Could you check a few things on this drawing? It's one solid part, dimensions in mm from its lowest x, y, z. A direction names the side the tool comes from. Give positions to 0.01 mm unless a question says otherwise; leave off trailing zeros. Order: outer loops, then holes, each group sorted by start corner. A loop starts at its lowest first (then second) coordinate and runs counter-clockwise, first axis right, second up. Notation, with made-up numbers: (7.5, 60) -> (22.5, 60) arc R33 cw to (22.5, 91) -> close; hole circle Ø4 at (-38.5, -36). An arc over 180 degrees is marked (long way). Answer as CSV lines item,"result".
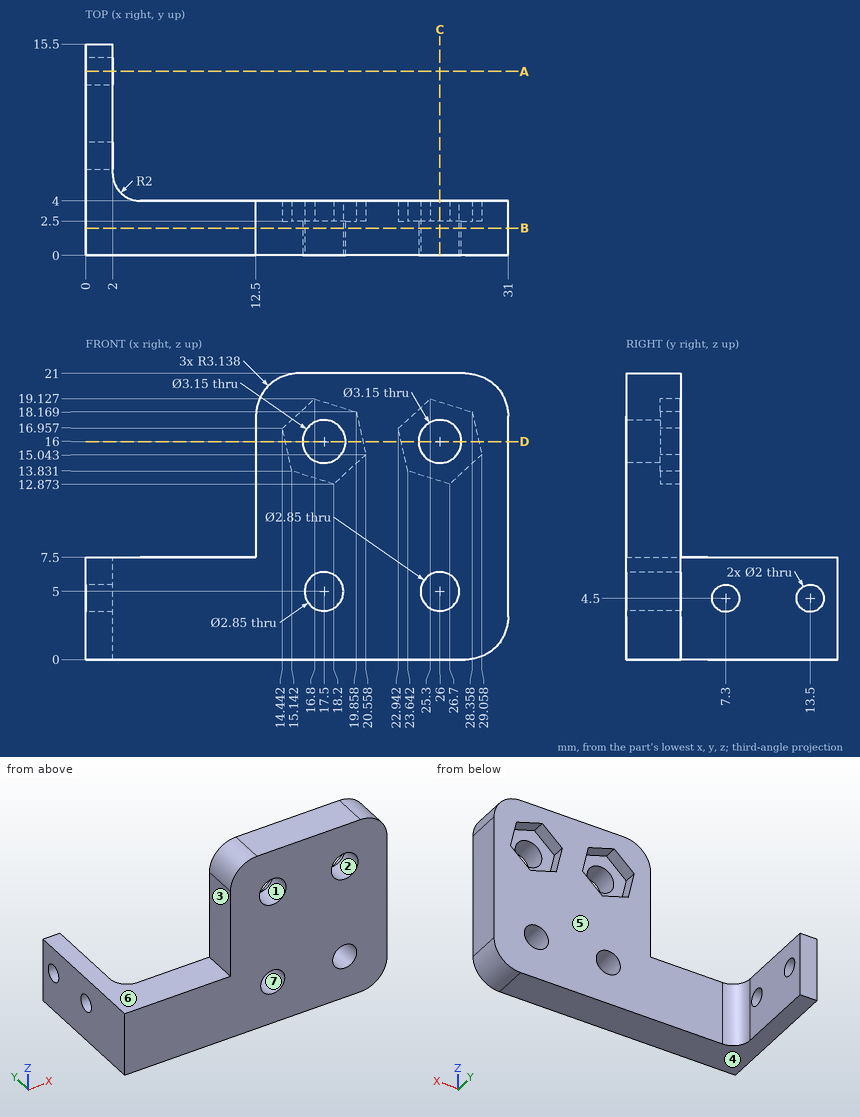
Item 1: Imagine slicing it at D-D, the plane z = 16. Please give me the cut outline in (x, y) (1 decimal).
Numbers:
outline,"(12.5, 0) -> (15.9, 0) -> (15.9, 2.5) -> (14.7, 2.5) -> (14.7, 4) -> (12.5, 4) -> close; (19.1, 0) -> (24.4, 0) -> (24.4, 2.5) -> (23.2, 2.5) -> (23.2, 4) -> (20.3, 4) -> (20.3, 2.5) -> (19.1, 2.5) -> close; (27.6, 0) -> (31, 0) -> (31, 4) -> (28.8, 4) -> (28.8, 2.5) -> (27.6, 2.5) -> close"
Item 2: Please list where these lines run through material, in increasing order: line 1 along Z through (x, y) = (17.5, 1.2) (1 decimal); line 2 along Z through (x, y) = (0.45, 7.3); line 3 along Z through (x, y) = (27, 1.25) (1 decimal).
Numbers:
line 1,"z = 0 to 3.6, 6.4 to 14.4, 17.6 to 21"
line 2,"z = 0 to 3.5, 5.5 to 7.5"
line 3,"z = 0 to 4, 6 to 14.8, 17.2 to 21"
Item 3: Imagine slicing it at B-B, the plane y = 2. Give the number of separate pieces and of enclosed holes in the cut face.
Numbers:
separate pieces,"1"
enclosed holes,"4"
Item 4: For pin 1 (5 mm diameter, centred on x = 15, z = 14.5, fed in from -Y); pin 2 (1.5 mm diameter, centred on x = 22, z = 18, fed in from +Y); pin 3 (1.2 mm diameter, centred on y = 1.5, z = 11, fed in from -X); pin 4 (2 mm diameter, centred on y = 12, z = 4, fed in from +X), each with a flat end and sliding along its axis, tell me the tip position at first contact or that it passes through.
Numbers:
pin 1,"stops at y = 0"
pin 2,"stops at y = 4"
pin 3,"stops at x = 12.5"
pin 4,"stops at x = 2"
Item 5: Imagine slicing it at C-C, the plane x = 26. Please give me the cut outline in (y, z) (1 decimal).
Numbers:
outline,"(0, 0) -> (4, 0) -> (4, 3.6) -> (0, 3.6) -> close; (0, 6.4) -> (4, 6.4) -> (4, 13.1) -> (2.5, 13.1) -> (2.5, 14.4) -> (0, 14.4) -> close; (0, 17.6) -> (2.5, 17.6) -> (2.5, 18.9) -> (4, 18.9) -> (4, 21) -> (0, 21) -> close"
Item 6: Imagine slicing it at A-A, the plane y = 13.5. Please give me the cut outline in (x, z).
Numbers:
outline,"(0, 0) -> (2, 0) -> (2, 3.5) -> (0, 3.5) -> close; (0, 5.5) -> (2, 5.5) -> (2, 7.5) -> (0, 7.5) -> close"
Item 7: For the marked faces 5, 6 and 7, which set-ups out of +Z, -Z, +X, -X, +Y, -Y let a thin tool reach every point of the face, with its end or its side?
Numbers:
face 5,"+Z, -Z, +X, +Y"
face 6,"+Z, -X, +Y, -Y"
face 7,"+Y, -Y"
Item 8: We'd pull the mould along Z, two halves only. Please class the marked faces 1, 2, 3 and 4: released by +Z, released by -Z, zero draft, split by the parting line, or undercut.
Numbers:
face 1,"undercut"
face 2,"undercut"
face 3,"zero draft"
face 4,"released by -Z"
